Work out the finished part from the listing and answer in its coordinate system (mm). Give positions to 0.01 mm unless a question says otherwise; leave off trailing zeros. Use a Markdown table: item, result. Add a question column.
Q1. Each of these flat-tipped pins is pushed along its axis until it touches: pin 1 Ø2.5 at (x, z) = (150, -34.25) entering from -Y; pin 2 Ø5 at (x, z) = (135, -24.25) entering from +Y. Where does it stop, or does it pass through?
Q2. Consider line 1 (X direction, y = 0.25, z = -24.25); line 2 (Z direction, x = 150, y = 0.4); line 3 (X direction, y = 0.5, z = -34.25). Determine where each line is inside the solid, lowest interval first.
Q3. For a pull along Z with two mould halves and no side action, classify faces 1 (the face through (-3, 0, -1)), 2 (the face through (147.985, 0.909, -32.965)) as pulls with the +Z half, pulls with the -Z half, needs draft (parallel to the pull), parting line crosses it, or undercut.
from build123d import *

# Parameters (mm, degrees)
SKETCH1_W                    = 404
SKETCH1_H                    = 112
BOSS_EXTRUDE1_DEPTH          = 3
CSK_FOR_M4_SFHCS1_AT_2_COUNT = 2
CSK_FOR_M4_SFHCS1_AT_2_PITCH = 30
CSK_FOR_M4_SFHCS1_AT_3_COUNT = 2
CSK_FOR_M4_SFHCS1_AT_3_PITCH = 18.027756377
LPATTERN1_COUNT              = 2
LPATTERN1_PITCH              = 240


with BuildPart() as part:
    # Sketch1 → Boss-Extrude1 (new body)
    with BuildSketch(Plane(origin=(0, 0, 0), x_dir=(1, 0, 0), z_dir=(0, 1, 0))):
        Rectangle(SKETCH1_W, SKETCH1_H)
    extrude(amount=BOSS_EXTRUDE1_DEPTH)

    # Sketch3 → CSK for M4 SFHCS1 (revolve, cut)
    with BuildSketch(Plane(origin=(120, 3, -34.25), x_dir=(0, 0, 1), z_dir=(1, 0, 0))):
        Polygon((0, 0), (0, 3), (2.25, 3), (2.25, 2.23), (4.48, 0), align=None)
    csk_for_m4_sfhcs1 = revolve(axis=Axis((120, 9.35, -34.25), (0, -1, 0)), mode=Mode.SUBTRACT)

    # CSK for M4 SFHCS1 at 2: CSK for M4 SFHCS1 ×2
    with Locations(*[(i * CSK_FOR_M4_SFHCS1_AT_2_PITCH, 0, 0) for i in range(1, CSK_FOR_M4_SFHCS1_AT_2_COUNT)]):
        add(csk_for_m4_sfhcs1, mode=Mode.SUBTRACT)

    # CSK for M4 SFHCS1 at 3: CSK for M4 SFHCS1 ×2
    with Locations(*[Vector(0.832050294337843, 0, 0.55470019622523) * (i * CSK_FOR_M4_SFHCS1_AT_3_PITCH) for i in range(1, CSK_FOR_M4_SFHCS1_AT_3_COUNT)]):
        add(csk_for_m4_sfhcs1, mode=Mode.SUBTRACT)

    # LPattern1: CSK for M4 SFHCS1 ×2
    with Locations(*[(-i * LPATTERN1_PITCH, 0, 0) for i in range(1, LPATTERN1_COUNT)]):
        add(csk_for_m4_sfhcs1, mode=Mode.SUBTRACT)

    # LPattern1 copy 1 sketch → LPattern1 copy 1 (revolve, cut)
    with BuildSketch(Plane(origin=(-90, 3, -34.25), x_dir=(0, 0, 1), z_dir=(1, 0, 0))):
        Polygon((0, 0), (0, 3), (2.25, 3), (2.25, 2.23), (4.48, 0), align=None)
    revolve(axis=Axis((-90, 9.35, -34.25), (0, -1, 0)), mode=Mode.SUBTRACT)

    # LPattern1 copy 2 sketch → LPattern1 copy 2 (revolve, cut)
    with BuildSketch(Plane(origin=(-105, 3, -24.25), x_dir=(0, 0, 1), z_dir=(1, 0, 0))):
        Polygon((0, 0), (0, 3), (2.25, 3), (2.25, 2.23), (4.48, 0), align=None)
    revolve(axis=Axis((-105, 9.35, -24.25), (0, -1, 0)), mode=Mode.SUBTRACT)


solid = part.part
Result set:
| question | item | result |
|---|---|---|
| 1 | pin 1 | passes through |
| 1 | pin 2 | stops at y = 1.02 |
| 2 | line 1 | x = -202 to -107.25, -102.75 to 132.75, 137.25 to 202 |
| 2 | line 2 | z = -56 to -36.5, -32 to 56 |
| 2 | line 3 | x = -202 to -122.25, -117.75 to -92.25, -87.75 to 117.75, 122.25 to 147.75, 152.25 to 202 |
| 3 | face 1 | needs draft |
| 3 | face 2 | undercut |
